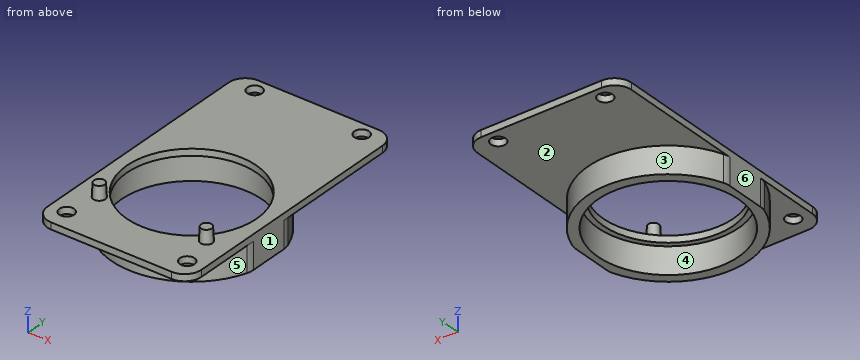
from build123d import *

# Parameters (mm, degrees)
SKETCH_1_W                = 23
SKETCH_1_H                = 40
EXTRUDE_1_DEPTH           = 1
SKETCH_2_R                = 9.7
CUT_EXTRUDE_1_DEPTH       = 28.083205128
FILLET_1_R                = 2.5
HOLE_WIZARD_M2_1_D        = 2.2
SKETCH_7_R                = 0.9
EXTRUDE_2_DEPTH           = 2
EXTRUDE_2_DRAFT           = 3
EXTRUDE_2_PROFILE_2_DEPTH = 2
EXTRUDE_2_PROFILE_2_DRAFT = 3
SKETCH_8_R                = 10.5
EXTRUDE_3_DEPTH           = 4
FILLET_2_R                = 3


with BuildPart() as part:
    # 草图1 → 凸台-拉伸1 (new body)
    with BuildSketch(Plane.XY):
        with Locations((0, 4.5)):
            Rectangle(SKETCH_1_W, SKETCH_1_H)
    extrude(amount=EXTRUDE_1_DEPTH)

    # 草图2 → 切除-拉伸1 (cut, through all)
    with BuildSketch(Plane.XY.offset(1)):
        Circle(SKETCH_2_R)
    extrude(amount=-CUT_EXTRUDE_1_DEPTH, mode=Mode.SUBTRACT)

    # 圆角1
    fillet_1_edges = [part.edges().sort_by_distance(p)[0] for p in [
        (-11.5, 24.5, 0.5),
        (11.5, 24.5, 0.5),
        (11.5, -15.5, 0.5),
        (-11.5, -15.5, 0.5),
    ]]
    fillet(fillet_1_edges, radius=FILLET_1_R)

    # M2 间隙孔1 (through all)
    with Locations(Plane.XY.offset(1)):
        with Locations((-8, 22.5), (8, 22.5), (-9, -12.5), (9, -12.5)):
            Hole(HOLE_WIZARD_M2_1_D / 2)


with BuildPart() as extrude_2_tool:
    # 草图7 → 凸台-拉伸2 (with draft: the straight prism first)
    with BuildSketch(Plane.XY.offset(1)):
        with Locations((-8, -7.5)):
            Circle(SKETCH_7_R)
    extrude(amount=EXTRUDE_2_DEPTH)
    # 凸台-拉伸2: the draft: its side faces are tilted about the plane it starts from
    extrude_2_sides = [extrude_2_tool.faces().sort_by_distance(p)[0] for p in [
        (-8.9, -7.5, 2),
    ]]
    draft(extrude_2_sides, Plane.XY.offset(1), EXTRUDE_2_DRAFT)


with BuildPart() as part_1:
    add(part.part)

    # 凸台-拉伸2: add extrude_2_tool
    add(extrude_2_tool.part)


with BuildPart() as extrude_2_profile_2_tool:
    # 草图7 → 凸台-拉伸2 profile 2 (with draft: the straight prism first)
    with BuildSketch(Plane.XY.offset(1)):
        with Locations((8, -7.5)):
            Circle(SKETCH_7_R)
    extrude(amount=EXTRUDE_2_PROFILE_2_DEPTH)
    # 凸台-拉伸2 profile 2: the draft: its side faces are tilted about the plane it starts from
    extrude_2_profile_2_sides = [extrude_2_profile_2_tool.faces().sort_by_distance(p)[0] for p in [
        (7.1, -7.5, 2),
    ]]
    draft(extrude_2_profile_2_sides, Plane.XY.offset(1), EXTRUDE_2_PROFILE_2_DRAFT)


with BuildPart() as part_2:
    add(part_1.part)

    # 凸台-拉伸2 profile 2: add extrude_2_profile_2_tool
    add(extrude_2_profile_2_tool.part)

    # 草图8 → 凸台-拉伸3 (add)
    with BuildSketch(Plane(origin=(0, 0, 0), x_dir=(-1, 0, 0), z_dir=(0, 0, -1))):
        with BuildLine():
            Line((11.5, 3.4278273), (11.5, -3.4278273))
            ThreePointArc((11.5, -3.4278273), (0, -12), (-11.5, -3.4278273))
            Line((-11.5, -3.4278273), (-11.5, 3.4278273))
            ThreePointArc((-11.5, 3.4278273), (0, 12), (11.5, 3.4278273))
        make_face()
        Circle(SKETCH_8_R, mode=Mode.SUBTRACT)
    extrude(amount=EXTRUDE_3_DEPTH)

    # 圆角2
    fillet_2_edges = [part_2.edges().sort_by_distance(p)[0] for p in [
        (-11.5, 3.4278273, -2),
        (11.5, 3.4278273, -2),
        (11.5, -3.4278273, -2),
        (-11.5, -3.4278273, -2),
    ]]
    fillet(fillet_2_edges, radius=FILLET_2_R)


solid = part_2.part
Source: CAD feature listing. Evaluate the final solid. Frame: model axes, mm. Face numbers are marked on the shaded views. A direction names the side the tool comes from. Give positions to 0.01 mm unless a question says otherwise; leave off trailing zeros. Order: outer loops, then holes, each group sorted by start corner. A loop starts at its lowest first (then second) coordinate and runs counter-clockwise, first axis right, second up. Notation, with made-up numbers: (-4.75, 7.25) -> (36.25, 7.25) arc R25 ccw to (36.25, 30.25) -> close; hole circle Ø6 at (66.5, 58). An arc over 180 degrees is marked (long way). Write item = value, one per line.
Q1. Pin query (flat end, axial travel): pin 1 (1 mm diameter, centred on y = -11, z = -1.5, fed in from -X); pin 2 (3 mm diameter, centred on x = -8, y = 22.5, fed in from +Z); pin 3 (4 mm diameter, centred on x = -7, y = 1.5, fed in from +Z). Return the tip coordinate at first contact, or that it passes through.
Data:
pin_1 = -5.81
pin_2 = 1
pin_3 = through
Q2. Cut plane B-B, the plane x = 0. Output: boundary loops of the cut face in (y, z), and give its area (3 significant figures).
Data:
outline = (-15.5, 0) -> (-12, 0) -> (-12, -4) -> (-10.5, -4) -> (-10.5, 0) -> (-9.7, 0) -> (-9.7, 1) -> (-15.5, 1) -> close; (9.7, 0) -> (10.5, 0) -> (10.5, -4) -> (12, -4) -> (12, 0) -> (24.5, 0) -> (24.5, 1) -> (9.7, 1) -> close
area = 32.6 mm^2
Q3. Cut plane A-A, the plane z = -2. Output: boundary loops of the cut face in (x, y), and give its area (3 significant figures).
Data:
outline = (-11.5, -2.96) arc R3 ccw to (-11.33, -3.94) arc R12 ccw to (11.33, -3.94) arc R3 ccw to (11.5, -2.96) -> (11.5, 2.96) arc R3 ccw to (11.33, 3.94) arc R12 ccw to (-11.33, 3.94) arc R3 ccw to (-11.5, 2.96) -> close; hole circle Ø21 at (0, 0)
area = 101 mm^2
Q4. Cut plane C-C, the plane y = 22.5. Output: boundary loops of the cut face in (x, z), and give its area (3 significant figures).
Data:
outline = (-11.45, 0) -> (-9.1, 0) -> (-9.1, 1) -> (-11.45, 1) -> close; (-6.9, 0) -> (6.9, 0) -> (6.9, 1) -> (-6.9, 1) -> close; (9.1, 0) -> (11.45, 0) -> (11.45, 1) -> (9.1, 1) -> close
area = 18.5 mm^2
Q5. Set-up query: the marked faces 5 and 6. Return all of +Z, -Z, +X, -X, +Y, -Y with unobstructed straight access to the full face (end or side cutting, diameter ignored); none if empty.
Data:
face_5 = -Z, -Y
face_6 = +Z, -Z, -X, +Y, -Y
Q6. Pull-direction query (X, two-part tool) for the marked faces 1, 2, 3 and 4; classes: released by +X, released by -X, zero draft, split by the parting line, or undercut.
Data:
face_1 = released by +X
face_2 = zero draft
face_3 = split by the parting line
face_4 = undercut
Q7. Material intervals for line 1 (Y direction, x = 0, z = -2.1); line 2 (Y direction, x = 8, z = 0.35); line 3 (Z direction, x = -9.5, y = 13.5), sorted ascending. Write a range as from..to.
Data:
line_1 = -12..-10.5, 10.5..12
line_2 = -15.5..-12.96, -12.04..-5.49, 5.49..21.4, 23.6..24.5
line_3 = 0..1
Q8. Cut plane D-D, the plane y = -7.5. Output: boundary loops of the cut face in (x, z).
Data:
outline = (-11.5, 0) -> (-9.37, 0) -> (-9.37, -4) -> (-7.35, -4) -> (-7.35, 0) -> (-6.15, 0) -> (-6.15, 1) -> (-7.1, 1) -> (-7.2, 3) -> (-8.8, 3) -> (-8.9, 1) -> (-11.5, 1) -> close; (6.15, 0) -> (7.35, 0) -> (7.35, -4) -> (9.37, -4) -> (9.37, 0) -> (11.5, 0) -> (11.5, 1) -> (8.9, 1) -> (8.8, 3) -> (7.2, 3) -> (7.1, 1) -> (6.15, 1) -> close
